The figure shows three views and two pictorial views of one solid part (mm, origin at its lowest corner). Answer the questions. Round coordinates to 2 decimals unless told otherwise and drop trailing zeros. Loops run counter-clockwise (first coordinate to the right, second up) from the corner with the lowest first, then second, coordinate; pieces in that order, holes last. Notation, with made-up numbers: (4, 88) -> (10, 88) arc R20 ccw to (10, 120) -> close; hole circle Ø4 at (-23, -5.75). An arc over 180 degrees is marked (long way). Put each result on its own line as item: value.
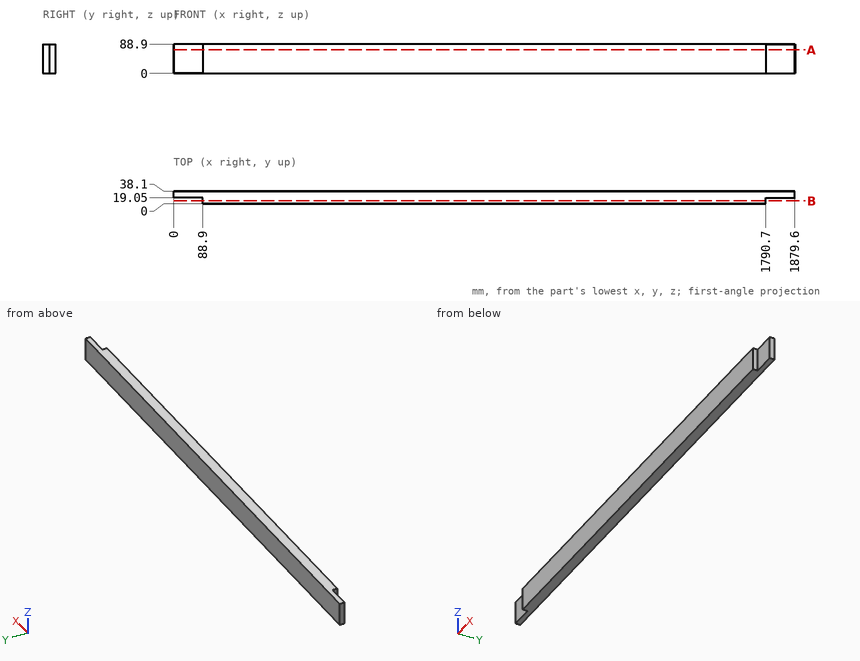
Item 1: Find the intervals of material crossed by line 1 along X through (y, z) = (12, 20), in increasing order.
Derived:
line 1: x = 88.9 to 1790.7
Item 2: The part is cut by section A-A (z = 71). Determine the outline of the cut face in (x, y), then the cut area to 3 significant figures.
Derived:
outline: (0, 19.05) -> (88.9, 19.05) -> (88.9, 0) -> (1790.7, 0) -> (1790.7, 19.05) -> (1879.6, 19.05) -> (1879.6, 38.1) -> (0, 38.1) -> close
area: 68,200 mm^2
Item 3: The part is cut by section B-B (y = 9.5). Determine the outline of the cut face in (x, z).
Derived:
outline: (88.9, 0) -> (1790.7, 0) -> (1790.7, 88.9) -> (88.9, 88.9) -> close
Item 4: Flat-ended cylindrical pins translate along their axes: pin 1 Ø3 at (x, z) = (735.5, 28.5) entering from -Y; pin 2 Ø4 at (y, z) = (10.5, 13) entering from -X. Find the tip coordinate at first contact, or state that the pin passes through.
Derived:
pin 1: stops at y = 0
pin 2: stops at x = 88.9
